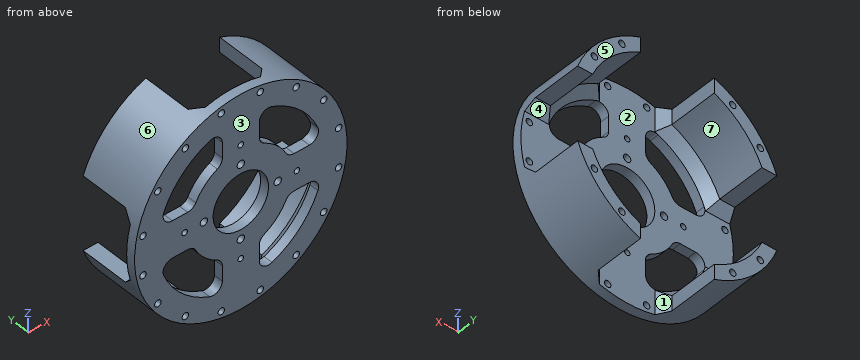
```python
from build123d import *

# Parameters (mm, degrees)
SKETCH1_R           = 57.5
BOSS_EXTRUDE1_DEPTH = 36.6
SKETCH2_R           = 50
CUT_EXTRUDE1_DEPTH  = 31.6
SKETCH3_R           = 2
SKETCH3_R_2         = 15
CUT_EXTRUDE2_DEPTH  = 31.8
SKETCH4_R           = 1.5
SKETCH4_R_2         = 1.75
CUT_EXTRUDE3_DEPTH  = 50
SKETCH9_W           = 40
SKETCH9_H           = 31.6
CUT_EXTRUDE4_DEPTH  = 72
CIRPATTERN1_COUNT   = 4
FILLET2_R           = 5
CHAMFER1_SIZE       = 5


with BuildPart() as part:
    # Sketch1 → Boss-Extrude1 (new body)
    with BuildSketch(Plane(origin=(0, 0, 0), x_dir=(1, 0, 0), z_dir=(0, 1, 0))):
        with Locations(Location((0, 0, 0), (0, 0, 270))):
            Circle(SKETCH1_R)
    extrude(amount=BOSS_EXTRUDE1_DEPTH)

    # Sketch2 → Cut-Extrude1 (cut)
    with BuildSketch(Plane(origin=(0, 36.6, 0), x_dir=(1, 0, 0), z_dir=(0, 1, 0))):
        with Locations(Location((0, 0, 0), (0, 0, 270))):
            Circle(SKETCH2_R)
    extrude(amount=-CUT_EXTRUDE1_DEPTH, mode=Mode.SUBTRACT)

    # Sketch3 → Cut-Extrude2 (cut)
    with BuildSketch(Plane.XZ):
        with BuildLine():
            Line((-10, 25.617376915), (-10, 43.874821937))
            ThreePointArc((-10, 43.874821937), (-31.819805153, 31.819805153), (-43.874821937, 10))
            Line((-43.874821937, 10), (-25.617376915, 10))
            ThreePointArc((-25.617376915, 10), (-19.445436483, 19.445436483), (-10, 25.617376915))
        make_face()
        with BuildLine():
            Line((25.617376915, 10), (43.874821937, 10))
            ThreePointArc((43.874821937, 10), (31.819805153, 31.819805153), (10, 43.874821937))
            Line((10, 43.874821937), (10, 25.617376915))
            ThreePointArc((10, 25.617376915), (19.445436483, 19.445436483), (25.617376915, 10))
        make_face()
        with BuildLine():
            ThreePointArc((10, -43.874821937), (31.819805153, -31.819805153), (43.874821937, -10))
            Line((43.874821937, -10), (25.617376915, -10))
            ThreePointArc((25.617376915, -10), (19.445436483, -19.445436483), (10, -25.617376915))
            Line((10, -25.617376915), (10, -43.874821937))
        make_face()
        with BuildLine():
            ThreePointArc((-43.874821937, -10), (-31.819805153, -31.819805153), (-10, -43.874821937))
            Line((-10, -43.874821937), (-10, -25.617376915))
            ThreePointArc((-10, -25.617376915), (-19.445436483, -19.445436483), (-25.617376915, -10))
            Line((-25.617376915, -10), (-43.874821937, -10))
        make_face()
        with Locations(Location((-20, 0, 0), (0, 0, 270))):
            Circle(SKETCH3_R)
        with Locations(Location((0, 0, 0), (0, 0, 270))):
            Circle(SKETCH3_R_2)
        with Locations(Location((0, 20, 0), (0, 0, 270))):
            Circle(SKETCH3_R)
        with Locations(Location((20, 0, 0), (0, 0, 270))):
            Circle(SKETCH3_R)
        with Locations(Location((0, -20, 0), (0, 0, 270))):
            Circle(SKETCH3_R)
    extrude(amount=-CUT_EXTRUDE2_DEPTH, mode=Mode.SUBTRACT)

    # Sketch4 → Cut-Extrude3 (cut)
    with BuildSketch(Plane.XZ):
        with Locations(Location((0, 30.405591591, 0), (0, 0, 270))):
            Circle(SKETCH4_R)
        with Locations(Location((30.405591591, 0, 0), (0, 0, 270))):
            Circle(SKETCH4_R)
        with Locations(Location((0, -30.405591591, 0), (0, 0, 270))):
            Circle(SKETCH4_R)
        with Locations(Location((-30.405591591, 0, 0), (0, 0, 270))):
            Circle(SKETCH4_R)
        with Locations(Location((-10.534877389, 52.962405142, 0), (0, 0, 270))):
            Circle(SKETCH4_R_2)
        with Locations(Location((10.534877389, 52.962405142, 0), (0, 0, 270))):
            Circle(SKETCH4_R_2)
        with Locations(Location((30.000792583, 44.899359064, 0), (0, 0, 270))):
            Circle(SKETCH4_R_2)
        with Locations(Location((44.899359064, 30.000792583, 0), (0, 0, 270))):
            Circle(SKETCH4_R_2)
        with Locations(Location((52.962405142, 10.534877389, 0), (0, 0, 270))):
            Circle(SKETCH4_R_2)
        with Locations(Location((52.962405142, -10.534877389, 0), (0, 0, 270))):
            Circle(SKETCH4_R_2)
        with Locations(Location((44.899359064, -30.000792583, 0), (0, 0, 270))):
            Circle(SKETCH4_R_2)
        with Locations(Location((30.000792583, -44.899359064, 0), (0, 0, 270))):
            Circle(SKETCH4_R_2)
        with Locations(Location((10.534877389, -52.962405142, 0), (0, 0, 270))):
            Circle(SKETCH4_R_2)
        with Locations(Location((-10.534877389, -52.962405142, 0), (0, 0, 270))):
            Circle(SKETCH4_R_2)
        with Locations(Location((-30.000792583, -44.899359064, 0), (0, 0, 270))):
            Circle(SKETCH4_R_2)
        with Locations(Location((-44.899359064, -30.000792583, 0), (0, 0, 270))):
            Circle(SKETCH4_R_2)
        with Locations(Location((-52.962405142, -10.534877389, 0), (0, 0, 270))):
            Circle(SKETCH4_R_2)
        with Locations(Location((-52.962405142, 10.534877389, 0), (0, 0, 270))):
            Circle(SKETCH4_R_2)
        with Locations(Location((-44.899359064, 30.000792583, 0), (0, 0, 270))):
            Circle(SKETCH4_R_2)
        with Locations(Location((-30.000792583, 44.899359064, 0), (0, 0, 270))):
            Circle(SKETCH4_R_2)
    extrude(amount=-CUT_EXTRUDE3_DEPTH, mode=Mode.SUBTRACT)

    # Sketch9 → Cut-Extrude4 (cut)
    with BuildSketch(Plane.XY):
        with Locations((0, 20.8)):
            Rectangle(SKETCH9_W, SKETCH9_H)
    cut_extrude4 = extrude(amount=-CUT_EXTRUDE4_DEPTH, mode=Mode.SUBTRACT)

    # CirPattern1: Cut-Extrude4 ×4 about axis
    cirpattern1_axis = Axis((0, 0, 0), (0, 1, 0))
    for i in range(1, CIRPATTERN1_COUNT):
        add(cut_extrude4.rotate(cirpattern1_axis, i * 360 / CIRPATTERN1_COUNT), mode=Mode.SUBTRACT)

    # Fillet2
    fillet2_edges = [part.edges().sort_by_distance(p)[0] for p in [
        (43.874821937, 2.5, 10),
        (25.617376915, 2.5, 10),
        (10, 2.5, 25.617376915),
        (10, 2.5, 43.874821937),
        (10, 2.5, -43.874821937),
        (10, 2.5, -25.617376915),
        (25.617376915, 2.5, -10),
        (43.874821937, 2.5, -10),
        (-43.874821937, 2.5, -10),
        (-25.617376915, 2.5, -10),
        (-10, 2.5, -25.617376915),
        (-10, 2.5, -43.874821937),
        (-10, 2.5, 43.874821937),
        (-10, 2.5, 25.617376915),
        (-25.617376915, 2.5, 10),
        (-43.874821937, 2.5, 10),
    ]]
    fillet(fillet2_edges, radius=FILLET2_R)

    # Chamfer1
    chamfer1_edges = [part.edges().sort_by_distance(p)[0] for p in [
        (-35.355339059, 5, -35.355339059),
        (-20, 5, -49.867701791),
        (20, 5, -49.867701791),
        (-35.355339059, 5, 35.355339059),
        (35.355339059, 5, 35.355339059),
        (35.355339059, 5, -35.355339059),
        (-49.867701791, 5, 20),
        (20, 5, 49.867701791),
        (49.867701791, 5, -20),
        (49.867701791, 5, 20),
        (-20, 5, 49.867701791),
        (-49.867701791, 5, -20),
    ]]
    chamfer(chamfer1_edges, length=CHAMFER1_SIZE - 0.0001)  # a hair under: the kernel refuses the full size


solid = part.part
```
Input: part model. Units: mm. Frame: model coordinates. Face numbers are marked on the shaded views. A direction names the side the tool comes from. Round coordinates to 2 decimals unless told otherwise and drop trailing zeros. Loops run counter-clockwise (first coordinate to the right, second up) from the corner with the lowest first, then second, coordinate; pieces in that order, holes last.
1) Material intervals for line 1 (X direction, y = 3, z = 19.5); line 2 (Z direction, x = 44.5, y = 4); line 3 (Z direction, x = -41, y = 14), sorted ascending.
Ans:
line 1: x = -54.09 to -40.56, -19.39 to -1.94, 1.94 to 19.39, 40.56 to 54.09
line 2: z = -36.41 to -31.7, -28.3 to 28.3, 31.7 to 36.41
line 3: z = -40.31 to -28.62, 28.62 to 40.31
2) Section query D-D on x = -40. Count the separate pieces of the cut face and the enclosed holes in it, plus the area to 3 significant figures.
Ans:
separate pieces: 3
enclosed holes: 0
area: 1,080 mm2
3) Set-up query: the marked faces 1, 2, 3 and 4. Return all of +Z, -Z, +X, -X, +Y, -Y with unobstructed straight access to the full face (end or side cutting, diameter ignored); none if empty.
Ans:
face 1: +Z, -Z, +Y
face 2: +Y
face 3: +Z, -Z, +X, -X, -Y
face 4: +X, -X, +Y
4) Pull-direction query (X, two-part tool) for the marked faces 5, 6 and 7; classes: released by +X, released by -X, zero draft, split by the parting line, or undercut.
Ans:
face 5: zero draft
face 6: split by the parting line
face 7: undercut
5) Pin query (flat end, axial travel): pin 1 (2 mm diameter, centred on y = 13, z = 26, fed in from +X); pin 2 (6 mm diameter, centred on y = 22.5, z = 45, fed in from -X); pin 3 (4 mm diameter, centred on y = 22.5, z = -49, fed in from +X). Return the tip coordinate at first contact, or that it passes through.
Ans:
pin 1: stops at x = 51.78
pin 2: stops at x = -39.27
pin 3: stops at x = 33.12
6) Section query A-A on z = 0. Return the cut outline in (x, y), plus the area to 3 significant figures.
Ans:
outline: (-57.5, 0) - (-31.91, 0) - (-31.91, 5) - (-57.5, 5) - close; (-28.91, 0) - (-22, 0) - (-22, 5) - (-28.91, 5) - close; (-18, 0) - (-15, 0) - (-15, 5) - (-18, 5) - close; (15, 0) - (18, 0) - (18, 5) - (15, 5) - close; (22, 0) - (28.91, 0) - (28.91, 5) - (22, 5) - close; (31.91, 0) - (57.5, 0) - (57.5, 5) - (31.91, 5) - close
area: 355 mm2
7) Section query B-B on x = 0. Return the cut outline in (y, z).
Ans:
outline: (0, -57.5) - (5, -57.5) - (5, -31.91) - (0, -31.91) - close; (0, -28.91) - (5, -28.91) - (5, -22) - (0, -22) - close; (0, -18) - (5, -18) - (5, -15) - (0, -15) - close; (0, 15) - (5, 15) - (5, 18) - (0, 18) - close; (0, 22) - (5, 22) - (5, 28.91) - (0, 28.91) - close; (0, 31.91) - (5, 31.91) - (5, 57.5) - (0, 57.5) - close
8) Section query C-C on z = 48.5. Return the cut outline in (x, y), plus the area to 3 significant figures.
Ans:
outline: (-30.89, 0) - (30.89, 0) - (30.89, 36.6) - (20, 36.6) - (20, 10) - (15, 5) - (-15, 5) - (-20, 10) - (-20, 36.6) - (-30.89, 36.6) - close
area: 1,020 mm2
